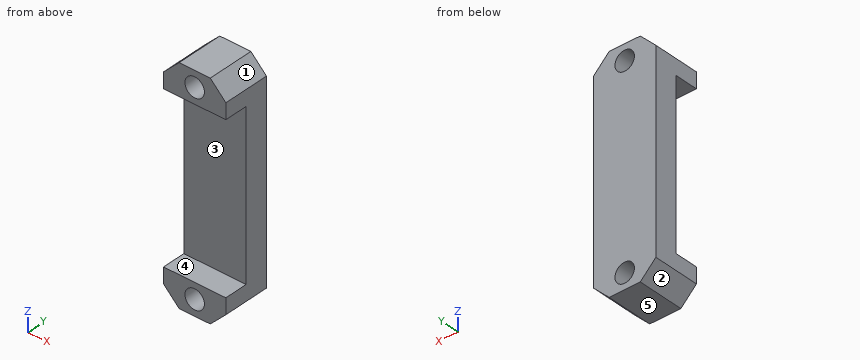
Autodesk Inventor part; units mm, degrees
ref_plane "YZ Plane" through (0, 0, 0) normal (1, 0, 0) x (0, 1, 0)
ref_plane "XZ Plane" through (0, 0, 0) normal (0, 1, 0) x (-1, 0, 0)
ref_plane "XY Plane" through (0, 0, 0) normal (0, 0, 1) x (1, 0, 0)
sketch "스케치1" plane through (0, 0, 0) normal (0, 1, 0) x (-1, 0, 0)
  line L0 (4, 14.5) -> (-4, 14.5)
  line L1 (-4, 14.5) -> (-4, -14.5)
  line L2 (-4, -14.5) -> (4, -14.5)
  line L3 (4, -14.5) -> (4, 14.5)
  line L4 (4, 14.5) -> (-4, -14.5) construction
  line L5 (-4, 14.5) -> (4, -14.5) construction
  line L6 (4, 10.5) -> (-4, 10.5)
  line L7 (0, 0) -> (3.2228, 0)
  line L8 (4, -10.5) -> (-4, -10.5)
  circle A0 centre (0, 12.5) radius 1.25
  circle A1 centre (0, -12.5) radius 1.25
  point P0 (4, -10.5)
  point P1 (-4, -10.5)
  dimension "d0" = 8
  dimension "d1" = 29
  dimension "d2" = 4
  dimension "d3" = 2.5
  dimension "d4" = 2
extrude "돌출1" add sketch "스케치1" against normal blind 3 contours L3 L6 L1 L0 | L3 L2 L1 L8
extrude "돌출2" add sketch "스케치1" along normal blind 3
chamfer "모따기1" distance 2 angle 45 4 edges at (4, 0, -14.5) (4, 0, 14.5) (-4, 0, 14.5) (-4, 0, -14.5)
properties part number "스텝모터 드라이버 홀더"
Part model, mm, in its own coordinate system. Face numbers are marked on the shaded views. A direction names the side the tool comes from. Round coordinates to 2 decimals unless told otherwise and drop trailing zeros. Order: outer loops, then holes, each group sorted by start corner. A loop starts at its lowest first (then second) coordinate and runs counter-clockwise, first axis right, second up. Notation, with made-up numbers: M 24.25,-8.5 L 77.25,-8.5 A33 ccw 77.25,22.5 Z; hole C -34,8.5 d11. An arc over 180 degrees is marked long. Answer in a Markdown table with one row per item. Add a question column.
Q1. 3-axis set-ups, long thin cutter, end or side, ignore diameter. For the marked faces 4 and 5: which of +Z, -Z, +X, -X, +Y, -Y reach the whole face in a straight line?
Q2. Cut at D-D on x = 0. Give the cut face in (y, z).
Q3. Mould opens along Z. For the marked faces 1, 2 and 3 say: +Z half, -Z half, draft (parallel to the pull), parting line (faces both ways), or undercut.
Q4. Wall check: L1, parallel to Z at x = 0, y = -1.5; L2, parallel to Z at x = 0, y = 1.8; L3, parallel to Y at x = -3, z = -5.5. Give the ranges that are in metal, low to high. Write a range as from..to.
Q5. Cut at B-B on y = 0.85. Give the cut face in (x, z).
Q6. Pin check, flat tip, straight feed: pin 1 (2.5 mm diameter, centred on x = -0.5, z = -5, fed in from -Y). Stop position of the tip, or through.
Q7. Cut at C-C on x = 2.25. Give the cut face in (y, z).
Q8. Cut at A-A on y = -1.7. Give the cut face in (x, z).
Established:
| question | item | result |
|---|---|---|
| 1 | face 4 | +X, -X, -Y |
| 1 | face 5 | -Z, +X, -X, +Y, -Y |
| 2 | outline | M -3,-14.5 L 3,-14.5 L 3,-13.75 L -3,-13.75 Z; M -3,-11.25 L 3,-11.25 L 3,11.25 L -3,11.25 L -3,10.5 L 0,10.5 L 0,-10.5 L -3,-10.5 Z; M -3,13.75 L 3,13.75 L 3,14.5 L -3,14.5 Z |
| 3 | face 1 | +Z half |
| 3 | face 2 | -Z half |
| 3 | face 3 | undercut |
| 4 | L1 | z = -14.5..-13.75, -11.25..-10.5, 10.5..11.25, 13.75..14.5 |
| 4 | L2 | z = -14.5..-13.75, -11.25..11.25, 13.75..14.5 |
| 4 | L3 | y = 0..3 |
| 5 | outline | M -4,-12.5 L -2,-14.5 L 2,-14.5 L 4,-12.5 L 4,12.5 L 2,14.5 L -2,14.5 L -4,12.5 Z; hole C 0,-12.5 d2.5; hole C 0,12.5 d2.5 |
| 6 | pin 1 | stops at y = 0 |
| 7 | outline | M -3,-14.25 L 3,-14.25 L 3,14.25 L -3,14.25 L -3,10.5 L 0,10.5 L 0,-10.5 L -3,-10.5 Z |
| 8 | outline | M -4,-12.5 L -2,-14.5 L 2,-14.5 L 4,-12.5 L 4,-10.5 L -4,-10.5 Z; M -4,10.5 L 4,10.5 L 4,12.5 L 2,14.5 L -2,14.5 L -4,12.5 Z; hole C 0,-12.5 d2.5; hole C 0,12.5 d2.5 |
